```python
from build123d import *

# Parameters (mm, degrees)
F0_R     = 22.622596
F1_DEPTH = 164.338
F2_R     = 11.902986
F3_DEPTH = 252.222
F4_R     = 11.692144
F5_DEPTH = 293.624
F6_R     = 20.169753
F7_DEPTH = 125.222
F8_R     = 14.537522
F9_DEPTH = 184.912


with BuildPart() as f1:
    # F0 (on Right) → F1 (new body)
    with BuildSketch(Plane.YZ):
        Circle(F0_R)
    extrude(amount=F1_DEPTH)

    # F2 (on Front) → F3 (join)
    with BuildSketch(Plane.XZ):
        Circle(F2_R)
    extrude(amount=F3_DEPTH)

    # F4 (on Front) → F5 (join)
    with BuildSketch(Plane.XZ):
        with Locations((129.934579, -13.058762)):
            Circle(F4_R)
    extrude(amount=F5_DEPTH)

    # F6 (on Top) → F7 (join)
    with BuildSketch(Plane.XY):
        Circle(F6_R)
    extrude(amount=F7_DEPTH)

    # F8 (on Front) → F9 (join)
    with BuildSketch(Plane.XZ):
        Circle(F8_R)
    extrude(amount=F9_DEPTH)


solid = f1.part
```
Model file for the job. Use its own axes, mm. A direction names the side the tool comes from. Give positions to 0.01 mm unless a question says otherwise; leave off trailing zeros. Write each loop counter-clockwise with the first axis right and the second up, starting at its lowest first coordinate (ties: lowest second). Pieces come first, ordered by that corner, then holes. Notation, with made-up numbers: M 8,28 L 13,28 A17 cw 13,55 Z; hole C 34,-10.5 d2. An arc over 180 degrees is marked long. Use a Markdown table: item, result.
1) Tool access for faces 5 (the flat face through (0, -252.222, 0)), 6 (the cylindrical face through (-20.15, 0.89, 61.73)), 7 (the cylindrical face through (81.02, 20.9, -8.66)), 8 (the flat face through (-5, -184.912, -11)), 9 (the flat face through (-10, 7, 0)): list every direction of +Z, -Z, +X, -X, +Y, -Y with a clear straight run to the whole face (end or side of a thin tool).
Responses:
| item | result |
|---|---|
| face 5 | +Z, -Z, -X, -Y |
| face 6 | +Z |
| face 7 | none |
| face 8 | -Y |
| face 9 | -Z, -X, +Y |
2) Cut at C-C (z = 36). List the corners of the cut face in (x, y), and give its area (3 significant figures).
Responses:
| item | result |
|---|---|
| outline | C 0,0 d40.34 |
| area | 1,280 mm2 |
3) Pull direction X, two halves, no side cores. Call faces 1 (the flat face through (0, 7, -11)), 2 (the cylindrical face through (11.35, -218.1, 3.58)), 3 (the cylindrical face through (-3.151, -91.162, -14.192)), 4 (the flat face through (130, -293.624, -13)): +X half, -X half, draft (parallel to the pull), parting line (faces both ways), or undercut.
Responses:
| item | result |
|---|---|
| face 1 | -X half |
| face 2 | undercut |
| face 3 | undercut |
| face 4 | draft |
4) Drill centre lines: line 1 (Y direction, x = 31, z = 1.5); line 2 (X direction, y = -257.5, z = -14); line 3 (X direction, y = -103, z = 0.5). Where is each one in solid material? Low to high. Write a range as from..to.
Responses:
| item | result |
|---|---|
| line 1 | y = -22.57..22.57 |
| line 2 | x = 118.28..141.59 |
| line 3 | x = -14.53..14.53 |
5) Cut at B-B (x = 128). List the corners of the cut face in (y, z), and give its area (3 significant figures).
Responses:
| item | result |
|---|---|
| outline | M -293.62,-24.59 L 0,-24.59 L 0,-22.62 A22.62 ccw long -22.57,-1.53 L -293.62,-1.53 Z |
| area | 8,010 mm2 |
6) Cut at D-D (x = 103). List the corners of the cut face in (y, z), and give its area (3 significant figures).
Responses:
| item | result |
|---|---|
| outline | C 0,0 d45.25 |
| area | 1,610 mm2 |
7) Pin check, flat tips, straight feed: pin 1 (1 mm diameter, centred on x = 47, z = -7, fed in from +Y); pin 2 (1.1 mm diameter, centred on x = 129.5, z = -23.5, fed in from +Y); pin 3 (6 mm diameter, centred on x = -8, y = 0.5, fed in from -Z). Stop position of each tip, or through.
Responses:
| item | result |
|---|---|
| pin 1 | stops at y = 21.67 |
| pin 2 | stops at y = 0 |
| pin 3 | stops at z = -13.64 |
8) Cut at A-A (y = -61). List the corners of the cut face in (x, z), and give its area (3 significant figures).
Responses:
| item | result |
|---|---|
| outline | C 0,0 d29.08; C 129.93,-13.06 d23.38 |
| area | 1,090 mm2 |
